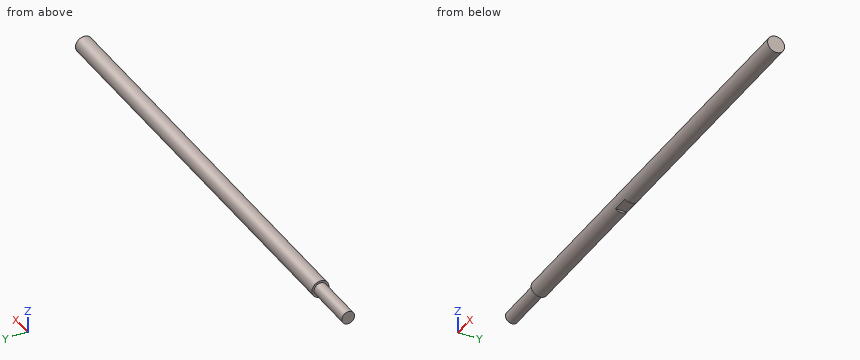
```python
from build123d import *

# Parameters (mm, degrees)
SKETCH3_W               = 25.4
SKETCH3_H               = 3.175
CUT_EXTRUDE1_DEPTH      = 725.12277274
CUT_EXTRUDE1_DEPTH_BACK = 725.12277274


with BuildPart() as part:
    # Sketch2 → Revolve1 (revolve)
    with BuildSketch(Plane(origin=(0, 0, 0), x_dir=(1, 0, 0), z_dir=(0, 1, 0)), mode=Mode.PRIVATE) as revolve1_sk:
        Polygon((-723.9, 9.525), (-723.9, 0), (0, 0), (0, 12.7), (-647.7, 12.7), (-647.7, 9.525), align=None)
    revolve(revolve1_sk.sketch.rotate(Axis((-723.9, 0, 0), (1, 0, 0)), 180), axis=Axis((-723.9, 0, 0), (1, 0, 0)))

    # Sketch3 → Cut-Extrude1 (cut, two sides)
    with BuildSketch(Plane(origin=(0, 0, 0), x_dir=(1, 0, 0), z_dir=(0, 1, 0))) as cut_extrude1_sk:
        with Locations((-411.48, 11.1125)):
            Rectangle(SKETCH3_W, SKETCH3_H)
    extrude(amount=CUT_EXTRUDE1_DEPTH, mode=Mode.SUBTRACT)
    extrude(cut_extrude1_sk.sketch, amount=-CUT_EXTRUDE1_DEPTH_BACK, mode=Mode.SUBTRACT)


solid = part.part
```
For this review, take the finished solid that the model builds, in its own axes (mm). Coordinates: 2 decimals unless noted, no trailing zeros. Loops run counter-clockwise (first coordinate to the right, second up) from the corner with the lowest first, then second, coordinate; pieces in that order, holes last. Notation, with made-up numbers: (23.25, -28) -> (77.25, -28) arc R30 cw to (77.25, -1) -> close; hole circle Ø10 at (-4.75, 2.25). An arc over 180 degrees is marked (long way). Return JSON: item names as keys, results as strings. Group by question number.
(1) Consider section D-D, the plane x = -469.5. Give the boundary of the cut face in (y, z).
(2) Consider section B-B, the plane y = 0. Give the boundary of the cut face in (x, z) (3 decimals), plus the area to 3 significant figures.
(3) For pin 1 Ø5 at (y, z) = (-9.5, -3) entering from -X; pin 2 Ø1 at (x, y) = (-287, -1) entering from +Z; pin 3 Ø6 at (x, y) = (-413.5, -7.5) entering from -Z (3 decimals); pin 4 Ø2 at (x, y) = (-379.5, 8) entering from -Z, all flat-tipped, find the tip position at first contact; note any pin that passes through.
(4) Consider section C-C, the plane x = -662.5. Give the boundary of the cut face in (y, z) (3 decimals), plus the area to 3 significant figures.
(5) To check wall thickness, follow L1, parallel to Y at x = -597.5, z = 0.75; L2, parallel to X at y = 10, z = 6; L3, parallel to Y at x = -523, z = -9.5. State the ranges of each line that lie inside material, in increasing order.
(6) Consider section A-A, the plane z = 0. Give the boundary of the cut face in (x, y) (3 decimals).
Results below:
{
 "1": {"outline": "circle Ø25.4 at (0, 0)"},
 "2": {"outline": "(-723.9, -9.525) -> (-647.7, -9.525) -> (-647.7, -12.7) -> (-424.18, -12.7) -> (-424.18, -9.525) -> (-398.78, -9.525) -> (-398.78, -12.7) -> (0, -12.7) -> (0, 12.7) -> (-647.7, 12.7) -> (-647.7, 9.525) -> (-723.9, 9.525) -> close", "area": "17,800 mm2"},
 "3": {"pin 1": "stops at x = -723.9", "pin 2": "stops at z = 12.69", "pin 3": "stops at z = -9.525", "pin 4": "stops at z = -10.6"},
 "4": {"outline": "circle Ø19.05 at (0, 0)", "area": "285 mm2"},
 "5": {"L1": "y = -12.68 to 12.68", "L2": "x = -647.7 to 0", "L3": "y = -8.43 to 8.43"},
 "6": {"outline": "(-723.9, -9.525) -> (-647.7, -9.525) -> (-647.7, -12.7) -> (0, -12.7) -> (0, 12.7) -> (-647.7, 12.7) -> (-647.7, 9.525) -> (-723.9, 9.525) -> close"}
}
